Check sheet for the drawn part. Datum: minimum x, y, z corner. Units: mm. Coordinates: 2 decimals unless noted, no trailing zeros. Loops run counter-clockwise (first coordinate to the right, second up) from the corner with the lowest first, then second, coordinate; pieces in that order, holes last.
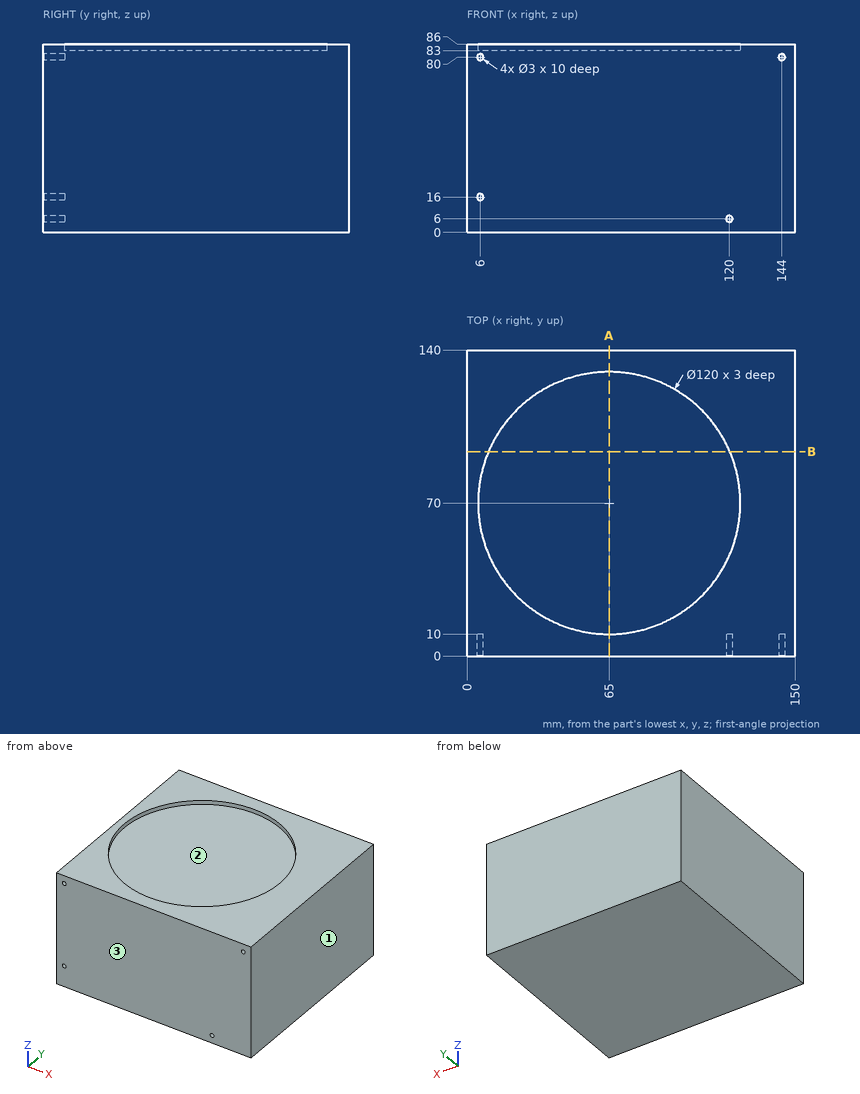
1) Mould release check, pull along X, two halves, no side actions. Record for the marked faces 1, 2 and 3: +X half, -X half, draft (parallel to the pull), parting line (faces both ways), or undercut.
Answer sheet:
face 1: +X half
face 2: undercut
face 3: draft
2) Depth check by flat-ended pin: pin 1 (1.8 mm diameter, centred on x = 120, z = 6, fed in from -Y); pin 2 (4 mm diameter, centred on x = 72, y = 68.5, fed in from +Z). Enter the tip coordinate at first touch or a pass-through.
Answer sheet:
pin 1: stops at y = 10
pin 2: stops at z = 83
3) Section check B-B on y = 93.5. Enter the section's corners in (x, z).
Answer sheet:
outline: (0, 0) - (150, 0) - (150, 86) - (120.21, 86) - (120.21, 83) - (9.79, 83) - (9.79, 86) - (0, 86) - close
4) Section check A-A on x = 65. Enter the section's corners in (y, z), plus the area to 3 significant figures.
Answer sheet:
outline: (0, 0) - (140, 0) - (140, 86) - (130, 86) - (130, 83) - (10, 83) - (10, 86) - (0, 86) - close
area: 11,700 mm2
5) Scan lines: line 1 (X direction, y = 7, z = 80); line 2 (Z direction, x = 144, y = 5.75); line 3 (Z direction, x = 72.5, y = 96). Record each from-to range of solid material in increasing order.
Answer sheet:
line 1: x = 0 to 4.5, 7.5 to 142.5, 145.5 to 150
line 2: z = 0 to 78.5, 81.5 to 86
line 3: z = 0 to 83
